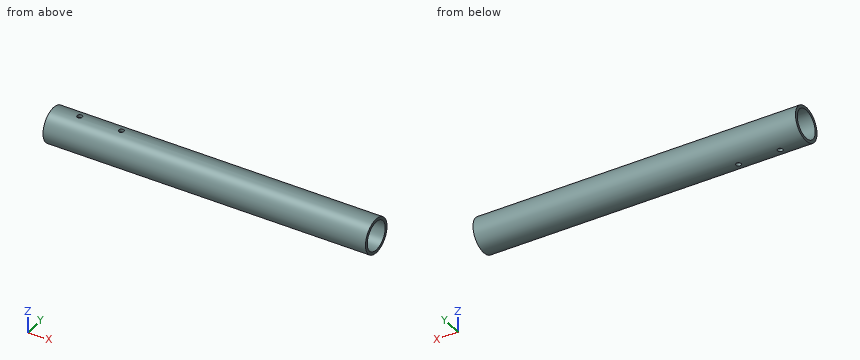
from build123d import *

# Parameters (mm, degrees)
SKETCH1_R                = 21.082
SKETCH1_R_2              = 17.526
BOSS_EXTRUDE1_DEPTH      = 196.85
BOSS_EXTRUDE1_DEPTH_BACK = 196.85
SKETCH2_R                = 3.175
CUT_EXTRUDE1_DEPTH       = 22.082
CUT_EXTRUDE1_DEPTH_BACK  = 22.082


with BuildPart() as part:
    # Sketch1 → Boss-Extrude1 (new body, two sides)
    with BuildSketch(Plane(origin=(0, 0, 0), x_dir=(0, 0, -1), z_dir=(1, 0, 0))) as boss_extrude1_sk:
        Circle(SKETCH1_R)
        Circle(SKETCH1_R_2, mode=Mode.SUBTRACT)
    extrude(amount=BOSS_EXTRUDE1_DEPTH)
    extrude(boss_extrude1_sk.sketch, amount=-BOSS_EXTRUDE1_DEPTH_BACK)

    # Sketch2 → Cut-Extrude1 (cut, two sides)
    with BuildSketch(Plane.XY) as cut_extrude1_sk:
        with Locations((-114.3, 0)):
            Circle(SKETCH2_R)
        with Locations((-165.1, 0)):
            Circle(SKETCH2_R)
    extrude(amount=CUT_EXTRUDE1_DEPTH, mode=Mode.SUBTRACT)
    extrude(cut_extrude1_sk.sketch, amount=-CUT_EXTRUDE1_DEPTH_BACK, mode=Mode.SUBTRACT)


solid = part.part
CAD build for the part. Positions are in the model's coordinates, mm. Give positions to 0.01 mm unless a question says otherwise; leave off trailing zeros. Write each loop counter-clockwise with the first axis right and the second up, starting at its lowest first coordinate (ties: lowest second). Pieces come first, ordered by that corner, then holes. Notation, with made-up numbers: (38, 33.25) - (55, 33.25) arc R28 cw to (55, 55.25) - close; hole circle Ø11 at (67, 75). An arc over 180 degrees is marked (long way). Answer as CSV lines item,"result".
Q1. Band-saw the part on C-C (x = 158.5). Give the cut face in (y, z).
Result set:
outline,"circle Ø42.16 at (0, 0); hole circle Ø35.05 at (0, 0)"
Q2. Flat gauge pins, fed straight in: pin 1 Ø12 at (x, y) = (-123, -14.5) entering from -Z; pin 2 Ø5 at (x, z) = (157.5, 16.5) entering from +Y; pin 3 Ø2 at (x, y) = (-139.5, 16) entering from -Z; pin 4 Ø5 at (x, y) = (-165.1, 0) entering from -Z. Where does each tip first touch, or does it go through?
Result set:
pin 1,"z = -19.29"
pin 2,"y = 15.76"
pin 3,"z = -14.81"
pin 4,"through"
Q3. Drill centre lines: line 1 (X direction, y = 0, z = -19) (3 decimals); line 2 (Z direction, x = -85, y = 0). Where is each one in solid material? Low to high. Write a range as from..to.
Result set:
line 1,"-196.85..-168.275, -161.925..-117.475, -111.125..196.85"
line 2,"-21.08..-17.53, 17.53..21.08"
Q4. Band-saw the part on B-B (y = -7.5). Give the cut face in (x, z), and give its area (3 significant figures).
Result set:
outline,"(-196.85, -19.7) - (196.85, -19.7) - (196.85, -15.84) - (-196.85, -15.84) - close; (-196.85, 15.84) - (196.85, 15.84) - (196.85, 19.7) - (-196.85, 19.7) - close"
area,"3,040 mm²"
Q5. Band-saw the part on A-A (z = 0). Give the cut face in (x, y).
Result set:
outline,"(-196.85, -21.08) - (196.85, -21.08) - (196.85, -17.53) - (-196.85, -17.53) - close; (-196.85, 17.53) - (196.85, 17.53) - (196.85, 21.08) - (-196.85, 21.08) - close"
